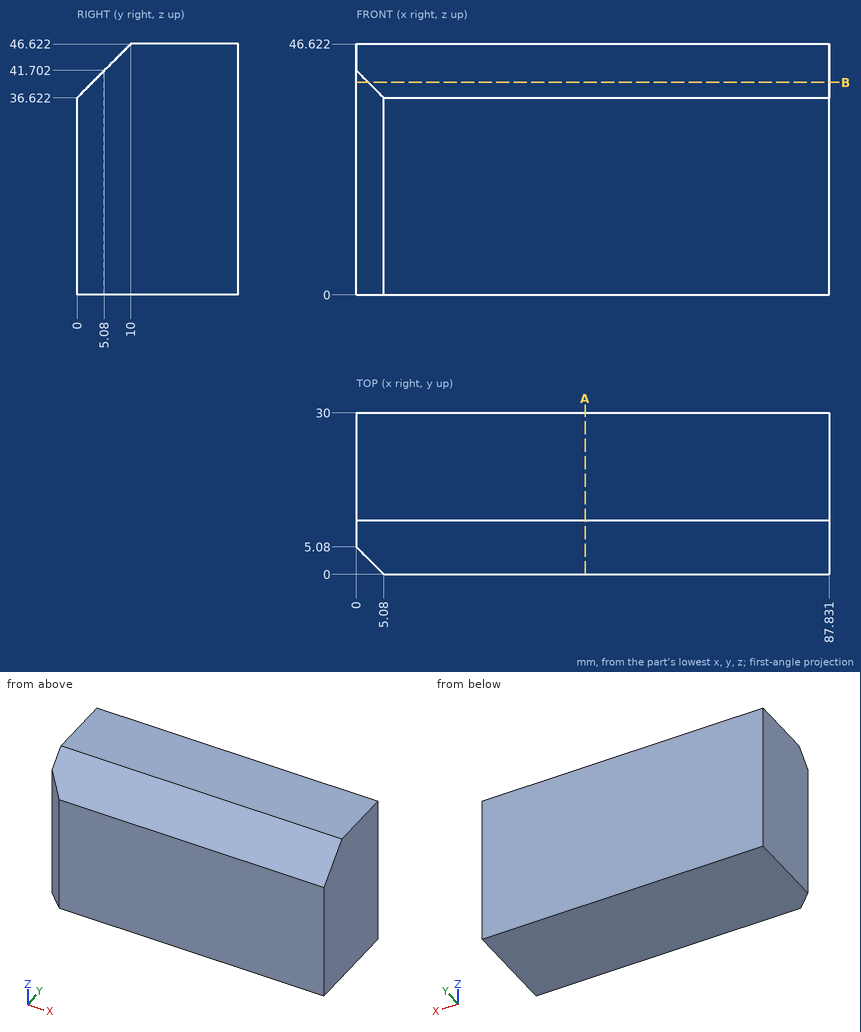
Study the drawing (mm; zero at the part's minimum x, y, z) and answer. Round coordinates to 2 decimals unless told otherwise and drop trailing zeros. Write each loop counter-clockwise with the first axis right and the second up, starting at its lowest first coordinate (ties: lowest second). Pieces come first, ordered by that corner, then holes. Notation, with made-up numbers: (20, 51.5) - (32, 51.5) arc R6 ccw to (32, 61.5) - close; hole circle Ø8 at (63, 85.5). An arc over 180 degrees is marked (long way). Return JSON: item names as keys, results as strings. Group by question number.
Q1. This flat-tipped pin is pushed along its axis until it touches: pin 1 Ø10 at (y, z) = (3.5, 36) entering from -X. Where does it stop, or does it pass through?
Q2. The part is cut by section A-A on x = 42.5. Write down the section's boundary in (y, z).
Q3. Find the intervals of material crossed by L1, parallel to Y at x = 74.5, z = 42 (1 decimal); L2, parallel to X at y = 1.75, z = 25; L3, parallel to Z at x = 36, y = 8 (1 decimal), in increasing order.
Q4. The part is cut by section B-B on z = 39.5. Write down the section's boundary in (x, y).
Solved:
{
 "1": {"pin 1": "x = 0"},
 "2": {"outline": "(0, 0) - (30, 0) - (30, 46.62) - (10, 46.62) - (0, 36.62) - close"},
 "3": {"L1": "5.4 to 30", "L2": "3.33 to 87.83", "L3": "0 to 44.6"},
 "4": {"outline": "(0, 5.08) - (2.2, 2.88) - (87.83, 2.88) - (87.83, 30) - (0, 30) - close"}
}
